Read the model definition and answer for the solid it produces. Units are mm, in the model's axes. A direction names the side the tool comes from. Round coordinates to 2 decimals unless told otherwise and drop trailing zeros. Write each loop counter-clockwise with the first axis right and the second up, starting at its lowest first coordinate (ties: lowest second). Pieces come first, ordered by that corner, then holes. Notation, with made-up numbers: (70, 38.25) -> (115, 38.25) arc R22 cw to (115, 72.25) -> close; hole circle Ø7 at (82.5, 12.5). An arc over 180 degrees is marked (long way). Return JSON: item names as keys, results as strings.
from build123d import *

# Parameters (mm, degrees)
F0_W     = 7.7216
F0_H     = 7.7216
F1_DEPTH = 4.826
F2_R     = 2.4511
F3_DEPTH = 1.778
F4_W     = 4.8768
F4_H     = 4.826
F5_DEPTH = 8.0518


with BuildPart() as f1:
    # F0 (on Top) → F1 (new body, symmetric)
    with BuildSketch(Plane.XY):
        Rectangle(F0_W, F0_H)
    extrude(amount=F1_DEPTH, both=True)

    # F2 (on face) → F3 (join)
    with BuildSketch(Plane.XY.offset(4.826)):
        Circle(F2_R)
    extrude(amount=F3_DEPTH)

    # F4 (on face) → F5 (cut)
    with BuildSketch(Plane(origin=(0, 0, -4.826), x_dir=(1, 0, 0), z_dir=(0, 0, -1))):
        Rectangle(F4_W, F4_H)
    extrude(amount=-F5_DEPTH, mode=Mode.SUBTRACT)


solid = f1.part
Item 1: A tool of negligible diameter and unlimited length cuts with its end or side. For faces 1 (the flat face through (-2, 2, 4.826)), 2 (the flat face through (2.438, 0, -1)), 3 (the flat face through (0, 0, 6.604)), from which of +Z, -Z, +X, -X, +Y, -Y can it reach the whole face along a straight path? Write none if from no direction.
Worked answers:
{"face 1": "+Z", "face 2": "-Z", "face 3": "+Z, +X, -X, +Y, -Y"}
Item 2: Section B-B (x = 0) is taken. Give the vertices of the cut face in (y, z).
Worked answers:
{"outline": "(-3.86, -4.83) -> (-2.41, -4.83) -> (-2.41, 3.23) -> (2.41, 3.23) -> (2.41, -4.83) -> (3.86, -4.83) -> (3.86, 4.83) -> (2.45, 4.83) -> (2.45, 6.6) -> (-2.45, 6.6) -> (-2.45, 4.83) -> (-3.86, 4.83) -> close"}
Item 3: Straight lines are drawn through the part: L1, parallel to Y at x = -0.75, z = 0; L2, parallel to X at y = 1.5, z = 1.5; L3, parallel to Z at x = 3, y = 3. For each, find the intervals that lie inside material, in ascending order. Write a range as [from, to].
Worked answers:
{"L1": "y = [-3.86, -2.41], [2.41, 3.86]", "L2": "x = [-3.86, -2.44], [2.44, 3.86]", "L3": "z = [-4.83, 4.83]"}
Item 4: A flat-ended cylindrical pin translates along its axis: pin 1 (1.4 mm diameter, centred on x = 1, y = -0.5, fed in from -Z). Find the tip coordinate at first contact, or state that the pin passes through.
Worked answers:
{"pin 1": "stops at z = 3.23"}
Item 5: For a pull along Y with two mould halves and no side action, classify faces 4 (the flat face through (0, -3.861, 0)), 5 (the flat face through (0, 3.861, 0)), 6 (the flat face through (0, 0, 3.226)) as released by +Y, released by -Y, zero draft, split by the parting line, or undercut.
Worked answers:
{"face 4": "released by -Y", "face 5": "released by +Y", "face 6": "undercut"}
Item 6: Section A-A (z = 0.5) is taken. Give the vertices of the cut face in (x, y).
Worked answers:
{"outline": "(-3.86, -3.86) -> (3.86, -3.86) -> (3.86, 3.86) -> (-3.86, 3.86) -> close; hole (-2.44, -2.41) -> (2.44, -2.41) -> (2.44, 2.41) -> (-2.44, 2.41) -> close"}
Item 7: Section D-D (y = 3) is taken. Give the vertices of the cut face in (x, z).
Worked answers:
{"outline": "(-3.86, -4.83) -> (3.86, -4.83) -> (3.86, 4.83) -> (-3.86, 4.83) -> close"}
Item 8: Section C-C (y = 0) is taken. Give the vertices of the cut face in (x, z).
Worked answers:
{"outline": "(-3.86, -4.83) -> (-2.44, -4.83) -> (-2.44, 3.23) -> (2.44, 3.23) -> (2.44, -4.83) -> (3.86, -4.83) -> (3.86, 4.83) -> (2.45, 4.83) -> (2.45, 6.6) -> (-2.45, 6.6) -> (-2.45, 4.83) -> (-3.86, 4.83) -> close"}
